```python
from build123d import *

# Parameters (mm, degrees)
F0_W      = 63.5
F0_H      = 50.8
F1_DEPTH  = 12.7
F3_DEPTH  = 12.7
F5_DEPTH  = 51.054
F6_W      = 12.7
F6_H      = 25.4
F7_DEPTH  = 25.4
F8_W      = 11.2009683429
F8_H      = 25.4
F9_DEPTH  = 12.7
F10_R     = 6.35
F11_DEPTH = 26.924


with BuildPart() as f1:
    # F0 (on Top) → F1 (new body)
    with BuildSketch(Plane.XY):
        with Locations((31.75, 25.4)):
            Rectangle(F0_W, F0_H)
    extrude(amount=F1_DEPTH)

    # F2 (on face) → F3 (join)
    with BuildSketch(Plane.XY.offset(12.7)):
        with BuildLine():
            Line((77.4110166286, 12.7), (77.4110166286, 38.1))
            ThreePointArc((77.4110166286, 38.1), (72.918152468, 47.1474711632), (63.5, 50.8))
            Line((63.5, 50.8), (63.5, 0))
            ThreePointArc((63.5, 0), (72.918152468, 3.6525288368), (77.4110166286, 12.7))
        make_face()
    extrude(amount=-F3_DEPTH)

    # F4 (on face) → F5 (join)
    with BuildSketch(Plane.XZ):
        Polygon((0, 38.1), (0, 12.7), (50.8, 12.7), (50.8, 25.4), (26.8990316571, 25.4), (26.8990316571, 50.8), (14.1990316571, 50.8), align=None)
    extrude(amount=-F5_DEPTH)

    # F6 (on face) → F7 (join)
    with BuildSketch(Plane.XY.offset(25.4)):
        with Locations((33.2490316571, 24.9606130317)):
            Rectangle(F6_W, F6_H)
    extrude(amount=F7_DEPTH)

    # F8 (on face) → F9 (join)
    with BuildSketch(Plane.XY.offset(25.4)):
        with Locations((45.1995158286, 24.9606130317)):
            Rectangle(F8_W, F8_H)
    extrude(amount=F9_DEPTH)

    # F10 (on face) → F11 (cut)
    with BuildSketch(Plane.YZ.offset(77.4110166286)):
        with Locations((25.4, 12.7)):
            Circle(F10_R)
    extrude(amount=-F11_DEPTH, mode=Mode.SUBTRACT)


solid = f1.part
```
Geometry check sheet. Reference: the model listing, model coordinates, mm. A direction names the side the tool comes from. Round coordinates to 2 decimals unless told otherwise and drop trailing zeros. Loops run counter-clockwise (first coordinate to the right, second up) from the corner with the lowest first, then second, coordinate; pieces in that order, holes last. Notation, with made-up numbers: M -37,35.5 L 0,35.5 A20 ccw 0,61.5 Z; hole C -3,20 d10. An arc over 180 degrees is marked long. Return JSON: item names as keys, results as strings. Group by question number.
(1) Section check C-C, the plane x = 28.5. Enter the section's corners in (y, z), and give its area (3 significant figures).
(2) Scan lines: line 1 along Z through (x, y) = (66, 25); line 2 along X through (y, z) = (44.5, 38); line 3 along Z through (x, y) = (53.5, 46). Record each from-to range of solid material in increasing order. Write a range as [from, to].
(3) Section check D-D, the plane y = 15.5. Enter the section's corners in (x, z).
(4) Section check B-B, the plane z = 33. Enter the section's corners in (x, y), and give its area (3 significant figures).
(5) Set-up check for faces 1 (the face through (64, 41, 12.7)), 2 (the face through (39, 44, 25.4)), 3 (the face through (39, 6, 25.4)): record each of +Z, -Z, +X, -X, +Y, -Y from which the full face is reachable in a straight line by a thin tool's end or side.
(6) Go/stop test with flat-tipped pins: pin 1 (7.5 mm diameter, centred on y = 26.5, z = 19.5, fed in from +X); pin 2 (7 mm diameter, centred on x = 35.5, z = 41, fed in from -Y); pin 3 (9.5 mm diameter, centred on x = 63, y = 41, fed in from +Z). Record where each tip stops, or that it passes through.
(7) Section check A-A, the plane y = 25.4. Enter the section's corners in (x, z), and give its area (3 significant figures).
(8) Mould release check, pull along Y, two halves, no side actions. Record for faces 4 (the face through (39.599, 25, 44)), 5 (the face through (64.137, 28.33, 7.066)), 6 (the face through (24, 0, 20)): pulls with the +Y half, pulls with the -Y half, needs draft (parallel to the pull), parting line crosses it, or undercut.
Data:
{
 "1": {"outline": "M 0,0 L 50.8,0 L 50.8,12.7 L 51.05,12.7 L 51.05,25.4 L 37.66,25.4 L 37.66,50.8 L 12.26,50.8 L 12.26,25.4 L 0,25.4 Z", "area": "1,940 mm²"},
 "2": {"line 1": "[0, 6.36]", "line 2": "[0, 26.9]", "line 3": "[0, 12.7]"},
 "3": {"outline": "M 0,0 L 77.41,0 L 77.41,12.7 L 50.8,12.7 L 50.8,38.1 L 39.6,38.1 L 39.6,50.8 L 14.2,50.8 L 0,38.1 Z"},
 "4": {"outline": "M 0,0 L 26.9,0 L 26.9,12.26 L 50.8,12.26 L 50.8,37.66 L 26.9,37.66 L 26.9,51.05 L 0,51.05 Z", "area": "1,980 mm²"},
 "5": {"face 1": "+Z, +X, +Y, -Y", "face 2": "+Z, +X, +Y", "face 3": "+Z, +X, -Y"},
 "6": {"pin 1": "x = 50.8", "pin 2": "y = 12.26", "pin 3": "z = 12.7"},
 "7": {"outline": "M 0,0 L 77.41,0 L 77.41,6.35 L 50.49,6.35 L 50.49,19.05 L 50.8,19.05 L 50.8,38.1 L 39.6,38.1 L 39.6,50.8 L 14.2,50.8 L 0,38.1 Z", "area": "2,510 mm²"},
 "8": {"face 4": "needs draft", "face 5": "undercut", "face 6": "pulls with the -Y half"}
}
